Geometry: final body of the model. Coordinates: model frame, mm. A direction names the side the tool comes from. Round coordinates to 2 decimals unless told otherwise and drop trailing zeros. Write each loop counter-clockwise with the first axis right and the second up, starting at its lowest first coordinate (ties: lowest second). Pieces come first, ordered by that corner, then holes. Notation, with made-up numbers: M -20,57 L 2,57 A22 cw 2,75 Z; hole C 30,30 d8. An arc over 180 degrees is marked long. Use one line per item in the form item = value. Start each with the question number.
Item 1: Ray query, probe 1 along X at (y, z) = (35.95, 15.5); probe 2 along X at (y, z) = (36, 15); probe 3 along X at (y, z) = (3, 0). Return the intervals inside material, ascending.
Item 2: Section query D-D (x = -6). Return loops of the section in (y, z).
Item 3: Section query B-B (y = 25.5). Return loops of the section in (x, z), and give its area (3 significant figures).
Item 4: Pull-direction query (X, two-part tool) for faces 6 (the flat face through (-5, 0, 2)), 7 (the cylindrical face through (-15.43, 35.53, 14)), 8 (the cylindrical face through (-10.74, 38.99, -2.38)); classes: pulls with the +X half, pulls with the -X half, needs draft (parallel to the pull), parting line crosses it, or undercut.
Item 5: Section query A-A (x = 0). Return loops of the section in (y, z).
Item 6: Section query C-C (z = 8). Return loops of the section in (x, y), and give its area (3 significant figures).
Item 7: Pin query (flat end, axial travel): pin 1 Ø0.9 at (x, z) = (-15.5, -16) entering from +Y; pin 2 Ø4.5 at (y, z) = (4.5, 24.5) entering from +X; pin 3 Ø6 at (y, z) = (50, 5) entering from +X. Return the tip coordinate at first contact, or that it passes through.
Item 8: Reachability of faces 1 (the cylindrical face through (15.57, 35.53, -17)), 2 (the flat face through (8.1, 5, 24)), 3 (the flat face through (-1.438, 52, 0)), 4 (the flat face through (-21, 19, 0)), 5 (the flat face through (1, 62, 0)) from +Z, -Z, +X, -X, +Y, -Y: full face, straight path, thin tool, end or side. Return the list, or none.
from build123d import *

# Parameters (mm, degrees)
SKETCH_1_W          = 42
SKETCH_1_H          = 42
EXTRUDE_1_DEPTH     = 38
SKETCH_2_R          = 11
EXTRUDE_2_DEPTH     = 2
SKETCH_3_R          = 2.5
EXTRUDE_3_DEPTH     = 22
SKETCH_5_W          = 16.2
SKETCH_5_H          = 9.2
EXTRUDE_4_DEPTH     = 5.5
SKETCH_6_R          = 1.5
CUT_EXTRUDE_1_DEPTH = 5
FILLET_1_R          = 5
SKETCH_7_R          = 4
CUT_EXTRUDE_2_DEPTH = 5
CUT_EXTRUDE_START   = -20
CUT_EXTRUDE_3_DEPTH = 20


with BuildPart() as part:
    # 草图1 → 凸台-拉伸1 (new body)
    with BuildSketch(Plane(origin=(0, 0, 0), x_dir=(1, 0, 0), z_dir=(0, 1, 0))):
        Rectangle(SKETCH_1_W, SKETCH_1_H)
    extrude(amount=EXTRUDE_1_DEPTH)

    # 草图2 → 凸台-拉伸2 (add)
    with BuildSketch(Plane(origin=(0, 38, 0), x_dir=(1, 0, 0), z_dir=(0, 1, 0))):
        with Locations(Location((0, 0, 0), (0, 0, 270))):
            Circle(SKETCH_2_R)
    extrude(amount=EXTRUDE_2_DEPTH)

    # 草图3 → 凸台-拉伸3 (add)
    with BuildSketch(Plane(origin=(0, 40, 0), x_dir=(1, 0, 0), z_dir=(0, 1, 0))):
        with Locations(Location((0, 0, 0), (0, 0, 270))):
            Circle(SKETCH_3_R)
    extrude(amount=EXTRUDE_3_DEPTH)

    # 草图5 → 凸台-拉伸4 (add)
    with BuildSketch(Plane.XY.offset(21)):
        with Locations((0, 4.6)):
            Rectangle(SKETCH_5_W, SKETCH_5_H)
    extrude(amount=EXTRUDE_4_DEPTH)

    # 草图6 → 切除-拉伸1 (cut)
    with BuildSketch(Plane(origin=(0, 38, 0), x_dir=(1, 0, 0), z_dir=(0, 1, 0))):
        with Locations(Location((-15.5, 15.5, 0), (0, 0, 270))):
            Circle(SKETCH_6_R)
        with Locations(Location((15.5, 15.5, 0), (0, 0, 270))):
            Circle(SKETCH_6_R)
        with Locations(Location((15.5, -15.5, 0), (0, 0, 270))):
            Circle(SKETCH_6_R)
        with Locations(Location((-15.5, -15.5, 0), (0, 0, 270))):
            Circle(SKETCH_6_R)
    extrude(amount=-CUT_EXTRUDE_1_DEPTH, mode=Mode.SUBTRACT)

    # 圆角1
    fillet_1_edges = [part.edges().sort_by_distance(p)[0] for p in [
        (21, 19, 21),
        (-21, 19, 21),
        (-21, 19, -21),
        (21, 19, -21),
    ]]
    fillet(fillet_1_edges, radius=FILLET_1_R)

    # 草图7 → 切除-拉伸2 (cut)
    with BuildSketch(Plane.XZ):
        with Locations(Location((0, 0, 0), (0, 0, 270))):
            Circle(SKETCH_7_R)
    extrude(amount=-CUT_EXTRUDE_2_DEPTH, mode=Mode.SUBTRACT)

    # 草图8 → 切除-拉伸3 (cut)
    with BuildSketch(Plane(origin=(0, 62, 0), x_dir=(1, 0, 0), z_dir=(0, 1, 0)).offset(CUT_EXTRUDE_START)):
        with BuildLine():
            Line((-1.438247, -2.044858324), (-1.438247, 2.044858324))
            ThreePointArc((-1.438247, 2.044858324), (-2.5, 0), (-1.438247, -2.044858324))
        make_face()
    extrude(amount=CUT_EXTRUDE_3_DEPTH, mode=Mode.SUBTRACT)


solid = part.part
Working result:
q1.probe_1 = -21 to -17, -14 to 14, 17 to 21
q1.probe_2 = -21 to -16.91, -14.09 to 14.09, 16.91 to 21
q1.probe_3 = -21 to -4, 4 to 21
q2.outline = M 0,-21 L 38,-21 L 38,-9.22 L 40,-9.22 L 40,9.22 L 38,9.22 L 38,21 L 9.2,21 L 9.2,26.5 L 0,26.5 Z
q3.outline = M -21,-16 A5 ccw -16,-21 L 16,-21 A5 ccw 21,-16 L 21,16 A5 ccw 16,21 L -16,21 A5 ccw -21,16 Z
q3.area = 1,740 mm²
q4.face_6 = needs draft
q4.face_7 = undercut
q4.face_8 = parting line crosses it
q5.outline = M 0,-21 L 38,-21 L 38,-11 L 40,-11 L 40,-2.5 L 62,-2.5 L 62,2.5 L 40,2.5 L 40,11 L 38,11 L 38,21 L 9.2,21 L 9.2,26.5 L 0,26.5 L 0,4 L 5,4 L 5,-4 L 0,-4 Z
q6.outline = M -21,0 L 21,0 L 21,38 L 7.55,38 L 7.55,40 L -7.55,40 L -7.55,38 L -21,38 Z
q6.area = 1,630 mm²
q7.pin_1 = 33
q7.pin_2 = 8.1
q7.pin_3 = 1.5
q8.face_1 = +Y
q8.face_2 = +Z, +X, +Y, -Y
q8.face_3 = +Z, -Z, -X, +Y
q8.face_4 = +Z, -Z, -X, +Y, -Y
q8.face_5 = +Z, -Z, +X, -X, +Y
